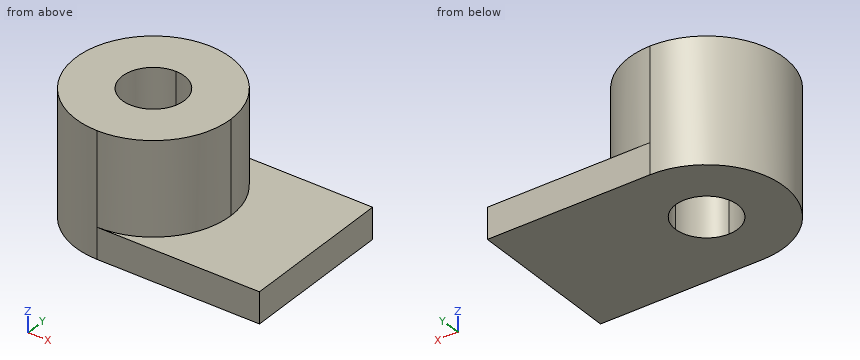
```python
from build123d import *

# Parameters (mm, degrees)
F1_DEPTH = 12.7
F2_DEPTH = 50.8


with BuildPart() as f1:
    # F0 (on Top) → F1 (new body)
    with BuildSketch(Plane.XY):
        with BuildLine():
            ThreePointArc((-1.538598, 0), (-10.837958, -22.45064), (-33.288598, -31.75))
            Line((-33.288598, -31.75), (33.288598, -31.75))
            Line((33.288598, -31.75), (33.288598, 31.75))
            Line((33.288598, 31.75), (-33.288598, 31.75))
            ThreePointArc((-33.288598, 31.75), (-10.837958, 22.45064), (-1.538598, 0))
        make_face()
        with BuildLine():
            ThreePointArc((-33.288598, 31.75), (-65.038598, 0), (-33.288598, -31.75))
            Line((-33.288598, -31.75), (-33.288598, -12.7))
            ThreePointArc((-33.288598, -12.7), (-45.988598, 0), (-33.288598, 12.7))
            Line((-33.288598, 12.7), (-33.288598, 31.75))
        make_face()
    extrude(amount=F1_DEPTH)

    # F0 (on Top) → F2 (join)
    with BuildSketch(Plane.XY):
        with BuildLine():
            Line((-33.288598, -12.7), (-33.288598, -31.75))
            ThreePointArc((-33.288598, -31.75), (-10.837958, -22.45064), (-1.538598, 0))
            ThreePointArc((-1.538598, 0), (-10.837958, 22.45064), (-33.288598, 31.75))
            Line((-33.288598, 31.75), (-33.288598, 12.7))
            ThreePointArc((-33.288598, 12.7), (-24.308342, 8.980256), (-20.588598, 0))
            ThreePointArc((-20.588598, 0), (-24.308342, -8.980256), (-33.288598, -12.7))
        make_face()
        with BuildLine():
            ThreePointArc((-33.288598, 31.75), (-65.038598, 0), (-33.288598, -31.75))
            Line((-33.288598, -31.75), (-33.288598, -12.7))
            ThreePointArc((-33.288598, -12.7), (-45.988598, 0), (-33.288598, 12.7))
            Line((-33.288598, 12.7), (-33.288598, 31.75))
        make_face()
    extrude(amount=F2_DEPTH)


solid = f1.part
```
Verification items for the finished model (mm, model axes). Coordinates: 2 decimals unless noted, no trailing zeros. Write each loop counter-clockwise with the first axis right and the second up, starting at its lowest first coordinate (ties: lowest second). Pieces come first, ordered by that corner, then holes. Notation, with made-up numbers: (50.5, 42) - (90.5, 42) arc R18 ccw to (90.5, 68) - close; hole circle Ø6 at (7.25, 26). An arc over 180 degrees is marked (long way). One line per question, with ' | ' between items. Start each with the question number.
1. Section check B-B (y = 6). Enter the section's corners in (x, z).
2. Section check D-D (y = -4.5). Enter the section's corners in (x, z), plus the area to 3 significant figures.
3. Gauge pin test, flat ends, axial feed: P1, Ø1, axis at x = -38.5, z = 31.5, coming from the -Y side; P2, Ø1.5, axis at y = -6.5, z = 24.5, coming from the -X side; P3, Ø6, axis at x = -11, z = 15, coming from the -Y side; P4, Ø2, axis at y = -9.5, z = 16, coming from the +X side. Record the tip position at first contact, or that the pin passes through.
4. Section check C-C (x = -42.5). Enter the section's corners in (y, z).
5. Material ranges on line 1 along Y through (x, z) = (-24, 47.5); line 2 along Y through (x, z) = (-22, 40); line 3 along X through (y, z) = (-9, 45.5), recorded low to high.
6. Section check A-A (z = 11). Enter the section's corners in (x, y), plus the area to 3 significant figures.
Computed values:
1) outline: (-64.47, 0) - (-44.48, 0) - (-44.48, 50.8) - (-64.47, 50.8) - close; (-22.1, 0) - (33.29, 0) - (33.29, 12.7) - (-2.11, 12.7) - (-2.11, 50.8) - (-22.1, 50.8) - close
2) outline: (-64.72, 0) - (-45.16, 0) - (-45.16, 50.8) - (-64.72, 50.8) - close; (-21.41, 0) - (33.29, 0) - (33.29, 12.7) - (-1.86, 12.7) - (-1.86, 50.8) - (-21.41, 50.8) - close | area: 2,430 mm²
3) P1: y = -31.4 | P2: x = -64.51 | P3: y = -31.75 | P4: x = -2.7
4) outline: (-30.38, 0) - (-8.74, 0) - (-8.74, 50.8) - (-30.38, 50.8) - close; (8.74, 0) - (30.38, 0) - (30.38, 50.8) - (8.74, 50.8) - close
5) line 1: -30.36 to -8.66, 8.66 to 30.36 | line 2: -29.68 to -5.82, 5.82 to 29.68 | line 3: -63.74 to -42.25, -24.33 to -2.84
6) outline: (-33.29, -31.75) - (33.29, -31.75) - (33.29, 31.75) - (-33.29, 31.75) arc R31.75 ccw to start; hole circle Ø25.4 at (-33.29, 0) | area: 5,300 mm²
